from build123d import *

# Parameters (mm, degrees)
F0_R     = 10
F1_DEPTH = 1.5
F2_DEPTH = 2


with BuildPart() as f1:
    # F0 (on Top) → F1 (new body)
    with BuildSketch(Plane.XY):
        with BuildLine():
            ThreePointArc((8.6602540378, 25.4), (0, 20.4), (-8.6602540378, 25.4))
            ThreePointArc((-8.6602540378, 25.4), (-10.5481894181, 6.09), (-26.327172275, -5.2))
            ThreePointArc((-26.327172275, -5.2), (-19.2561044632, -8.1289321881), (-16.327172275, -15.2))
            ThreePointArc((-16.327172275, -15.2), (-16.6679140122, -17.788190451), (-17.6669182372, -20.2))
            ThreePointArc((-17.6669182372, -20.2), (0, -12.18), (17.6669182372, -20.2))
            ThreePointArc((17.6669182372, -20.2), (17.6669182372, -10.2), (26.327172275, -5.2))
            ThreePointArc((26.327172275, -5.2), (10.5481894181, 6.09), (8.6602540378, 25.4))
        make_face()
        Circle(F0_R, mode=Mode.SUBTRACT)
        with BuildLine():
            ThreePointArc((4.2868257487, 27.925), (0, 25.45), (-4.2868257487, 27.925))
            Line((-4.2868257487, 27.925), (-8.6602540378, 25.4))
            ThreePointArc((-8.6602540378, 25.4), (0, 20.4), (8.6602540378, 25.4))
            Line((8.6602540378, 25.4), (4.2868257487, 27.925))
        make_face()
        with BuildLine():
            Line((-8.6602540378, 25.4), (-4.2868257487, 27.925))
            ThreePointArc((-4.2868257487, 27.925), (-1.2811542733, 35.1813328401), (4.95, 30.4))
            ThreePointArc((4.95, 30.4), (4.7813328401, 29.1188457267), (4.2868257487, 27.925))
            Line((4.2868257487, 27.925), (8.6602540378, 25.4))
            ThreePointArc((8.6602540378, 25.4), (9.6592582629, 27.811809549), (10, 30.4))
            ThreePointArc((10, 30.4), (-2.588190451, 40.0592582629), (-8.6602540378, 25.4))
        make_face()
        with BuildLine():
            Line((26.327172275, -10.25), (26.327172275, -5.2))
            ThreePointArc((26.327172275, -5.2), (17.6669182372, -10.2), (17.6669182372, -20.2))
            Line((17.6669182372, -20.2), (22.0403465263, -17.675))
            ThreePointArc((22.0403465263, -17.675), (22.0403465263, -12.725), (26.327172275, -10.25))
        make_face()
        with BuildLine():
            ThreePointArc((36.327172275, -15.2), (33.3982400869, -8.1289321881), (26.327172275, -5.2))
            Line((26.327172275, -5.2), (26.327172275, -10.25))
            ThreePointArc((26.327172275, -10.25), (29.8273508419, -11.6998214331), (31.277172275, -15.2))
            ThreePointArc((31.277172275, -15.2), (27.6083265483, -19.9813328401), (22.0403465263, -17.675))
            Line((22.0403465263, -17.675), (17.6669182372, -20.2))
            ThreePointArc((17.6669182372, -20.2), (28.9153627261, -24.8592582629), (36.327172275, -15.2))
        make_face()
        with BuildLine():
            ThreePointArc((-16.327172275, -15.2), (-19.2561044632, -8.1289321881), (-26.327172275, -5.2))
            Line((-26.327172275, -5.2), (-26.327172275, -10.25))
            ThreePointArc((-26.327172275, -10.25), (-22.8269937082, -11.6998214331), (-21.377172275, -15.2))
            ThreePointArc((-21.377172275, -15.2), (-21.5458394349, -16.4811542733), (-22.0403465263, -17.675))
            Line((-22.0403465263, -17.675), (-17.6669182372, -20.2))
            ThreePointArc((-17.6669182372, -20.2), (-16.6679140122, -17.788190451), (-16.327172275, -15.2))
        make_face()
        with BuildLine():
            Line((-26.327172275, -10.25), (-26.327172275, -5.2))
            ThreePointArc((-26.327172275, -5.2), (-34.9874263129, -20.2), (-17.6669182372, -20.2))
            Line((-17.6669182372, -20.2), (-22.0403465263, -17.675))
            ThreePointArc((-22.0403465263, -17.675), (-30.6139980238, -17.675), (-26.327172275, -10.25))
        make_face()
    extrude(amount=F1_DEPTH)

    # F0 (on Top) → F2 (join)
    with BuildSketch(Plane.XY):
        with BuildLine():
            ThreePointArc((3.4208003449, 28.425), (0, 26.45), (-3.4208003449, 28.425))
            Line((-3.4208003449, 28.425), (-4.2868257487, 27.925))
            ThreePointArc((-4.2868257487, 27.925), (0, 25.45), (4.2868257487, 27.925))
            Line((4.2868257487, 27.925), (3.4208003449, 28.425))
        make_face()
        with BuildLine():
            ThreePointArc((-3.4208003449, 28.425), (-1.0223352282, 34.2154070138), (3.95, 30.4))
            ThreePointArc((3.95, 30.4), (3.8154070138, 29.3776647718), (3.4208003449, 28.425))
            Line((3.4208003449, 28.425), (4.2868257487, 27.925))
            ThreePointArc((4.2868257487, 27.925), (4.7813328401, 29.1188457267), (4.95, 30.4))
            ThreePointArc((4.95, 30.4), (-1.2811542733, 35.1813328401), (-4.2868257487, 27.925))
            Line((-4.2868257487, 27.925), (-3.4208003449, 28.425))
        make_face()
        with BuildLine():
            Line((26.327172275, -11.25), (26.327172275, -10.25))
            ThreePointArc((26.327172275, -10.25), (22.0403465263, -12.725), (22.0403465263, -17.675))
            Line((22.0403465263, -17.675), (22.9063719301, -17.175))
            ThreePointArc((22.9063719301, -17.175), (22.9063719301, -13.225), (26.327172275, -11.25))
        make_face()
        with BuildLine():
            ThreePointArc((31.277172275, -15.2), (29.8273508419, -11.6998214331), (26.327172275, -10.25))
            Line((26.327172275, -10.25), (26.327172275, -11.25))
            ThreePointArc((26.327172275, -11.25), (29.1202440607, -12.4069282143), (30.277172275, -15.2))
            ThreePointArc((30.277172275, -15.2), (27.3495075032, -19.0154070138), (22.9063719301, -17.175))
            Line((22.9063719301, -17.175), (22.0403465263, -17.675))
            ThreePointArc((22.0403465263, -17.675), (27.6083265483, -19.9813328401), (31.277172275, -15.2))
        make_face()
        with BuildLine():
            ThreePointArc((-21.377172275, -15.2), (-22.8269937082, -11.6998214331), (-26.327172275, -10.25))
            Line((-26.327172275, -10.25), (-26.327172275, -11.25))
            ThreePointArc((-26.327172275, -11.25), (-23.5341004894, -12.4069282143), (-22.377172275, -15.2))
            ThreePointArc((-22.377172275, -15.2), (-22.5117652612, -16.2223352282), (-22.9063719301, -17.175))
            Line((-22.9063719301, -17.175), (-22.0403465263, -17.675))
            ThreePointArc((-22.0403465263, -17.675), (-21.5458394349, -16.4811542733), (-21.377172275, -15.2))
        make_face()
        with BuildLine():
            Line((-26.327172275, -11.25), (-26.327172275, -10.25))
            ThreePointArc((-26.327172275, -10.25), (-30.6139980238, -17.675), (-22.0403465263, -17.675))
            Line((-22.0403465263, -17.675), (-22.9063719301, -17.175))
            ThreePointArc((-22.9063719301, -17.175), (-29.74797262, -17.175), (-26.327172275, -11.25))
        make_face()
    extrude(amount=F2_DEPTH)


solid = f1.part
Read the model definition and answer for the solid it produces. Units are mm, in the model's axes. A direction names the side the tool comes from. Give positions to 0.01 mm unless a question says otherwise; leave off trailing zeros. Write each loop counter-clockwise with the first axis right and the second up, starting at its lowest first coordinate (ties: lowest second). Pieces come first, ordered by that corner, then holes. Notation, with made-up numbers: (2, 75.5) - (48, 75.5) arc R11 cw to (48, 82.5) - close; hole circle Ø6 at (84, 81). An arc over 180 degrees is marked (long way). Use CSV: the item, a comma, the result in double quotes. Start each with the question number.
(1) Find section C-C (y = 0). Give the vertices of the cut face in (x, z), plus the area to 3 significant figures.
(2) For faces 1 (the flat face through (-0.2, 10.2, 1.5)), 2 (the cylindrical face through (-2.17, -9.76, 0.74)), determine the directions among +Z, -Z, +X, -X, +Y, -Y from which every point of the face is accessible in a straight line to the end or side of a thin tool.
(3) Find section B-B (z = 0.75). Give the vertices of the cut face in (x, y) (3 decimals), plus the area to 3 significant figures.
(4) Find section D-D (y = -14). Give the vertices of the cut face in (x, z).
(5) Given P1, Ø6.5, axis at x = -26.33, y = -15.2, coming from the +Z side; P2, Ø12.5, axis at x = 0, y = 30.4, coming from the +Z side; P3, Ø1, axis at y = 21.5, z = 1, coming from the -X side, each flat-ended and moving along its own axis, determine where each tip first touches the part or whether it passes through.
(6) Find section A-A (x = 0). Give the vertices of the cut face in (y, z).
(7) Consider line 1 along X through (y, z) = (-15.2, 1.55); line 2 along X through (y, z) = (30.4, 0.65); line 3 along X through (y, z) = (-15.2, 1.2). Determine where each line is inside the solid, lowest interval first.
(8) Determine the mould class of faces 3 (the cylindrical face through (-0.28, -12.18, 0.74)), 4 (the flat face through (24, -19, 2)), 5 (the cylindrical face through (-10.41, 6.33, 0.74)), 6 (the cylindrical face through (10.69, 5.85, 0.74)) for opening direction X: +X half, -X half, draft (parallel to the pull), parting line (faces both ways), or undercut.
Findings below:
1,outline,"(-15.61, 0) - (-10, 0) - (-10, 1.5) - (-15.61, 1.5) - close; (10, 0) - (15.61, 0) - (15.61, 1.5) - (10, 1.5) - close"
1,area,"16.8 mm2"
2,face 1,"+Z"
2,face 2,"+Z, -Z"
3,outline,"(-26.327, -5.2) arc R10 ccw (long way) to (-17.667, -20.2) arc R23.469 cw to (17.667, -20.2) arc R10 ccw (long way) to (26.327, -5.2) arc R23.469 cw to (8.66, 25.4) arc R10 ccw (long way) to (-8.66, 25.4) arc R23.469 cw to start; hole circle Ø7.9 at (-26.327, -15.2); hole circle Ø20 at (0, 0); hole circle Ø7.9 at (0, 30.4); hole circle Ø7.9 at (26.327, -15.2)"
3,area,"1,440 mm2"
4,outline,"(-36.25, 0) - (-30.09, 0) - (-30.09, 2) - (-31.13, 2) - (-31.13, 1.5) - (-36.25, 1.5) - close; (-22.56, 0) - (-9.06, 0) - (-9.06, 1.5) - (-21.52, 1.5) - (-21.52, 2) - (-22.56, 2) - close; (9.06, 0) - (22.56, 0) - (22.56, 2) - (21.52, 2) - (21.52, 1.5) - (9.06, 1.5) - close; (30.09, 0) - (36.25, 0) - (36.25, 1.5) - (31.13, 1.5) - (31.13, 2) - (30.09, 2) - close"
5,P1,"through"
5,P2,"z = 2"
5,P3,"x = -7.78"
6,outline,"(-12.18, 0) - (-10, 0) - (-10, 1.5) - (-12.18, 1.5) - close; (10, 0) - (26.45, 0) - (26.45, 2) - (25.45, 2) - (25.45, 1.5) - (10, 1.5) - close; (34.35, 0) - (40.4, 0) - (40.4, 1.5) - (35.35, 1.5) - (35.35, 2) - (34.35, 2) - close"
7,line 1,"-31.28 to -30.28, -22.38 to -21.38, 21.38 to 22.38, 30.28 to 31.28"
7,line 2,"-10 to -3.95, 3.95 to 10"
7,line 3,"-36.33 to -30.28, -22.38 to -11.52, 11.52 to 22.38, 30.28 to 36.33"
8,face 3,"undercut"
8,face 4,"draft"
8,face 5,"-X half"
8,face 6,"+X half"
